from build123d import *

# Parameters (mm, degrees)
SKICA1_R               = 1.6
Z_KLADN_PLECH1_DEPTH   = 0.35
OHYB_START             = -2
OHYB_ZE_SKICI1_DEPTH   = 4
OHYB_ZE_SKICI1_2_DEPTH = 4


# Read off the part's stored shape, not the designer's step: Ohyb ze skici1
# Sheet-metal steps are written as plain solids
with BuildPart() as part:
    # Skica1 → Základní plech1 (new body)
    with BuildSketch(Plane(origin=(0, 0, 0), x_dir=(1, 0, 0), z_dir=(0, 1, 0))):
        with BuildLine():
            Line((6, 2), (13, 2))
            Line((13, 2), (13, -2))
            Line((13, -2), (6, -2))
            ThreePointArc((6, -2), (4.881966011, -2.263932023), (4, -3))
            ThreePointArc((4, -3), (-5, 0), (4, 3))
            ThreePointArc((4, 3), (4.881966011, 2.263932023), (6, 2))
        make_face()
        with Locations(Location((0, 0, 0), (0, 0, 270))):
            Circle(SKICA1_R, mode=Mode.SUBTRACT)
    extrude(amount=Z_KLADN_PLECH1_DEPTH)

    # Ohyb ze skici1 outline → Ohyb ze skici1 (cut)
    with BuildSketch(Plane.XY.offset(OHYB_START)):
        with BuildLine():
            ThreePointArc((7.3, 0.350000005), (7.728660709, 0.258514479), (8.082623799, 0))
            Line((8.082623799, 0), (13, 0))
            Line((13, 0), (13, 0.35))
            Line((13, 0.35), (7.3, 0.350000005))
        make_face()
    extrude(amount=OHYB_ZE_SKICI1_DEPTH, mode=Mode.SUBTRACT)

    # Ohyb ze skici1 2 outline → Ohyb ze skici1 2 (add)
    with BuildSketch(Plane.XY.offset(OHYB_START)):
        with BuildLine():
            Line((8.35, -5.025553214), (8.350000005, -0.700000005))
            ThreePointArc((8.350000005, -0.700000005), (8.280880984, -0.325336808), (8.082623799, 0))
            Line((8.082623799, 0), (7.3, 5e-09))
            ThreePointArc((7.3, 5e-09), (7.79497475, -0.20502525), (8.000000005, -0.7))
            Line((8.000000005, -0.7), (8, -5.025553214))
            Line((8, -5.025553214), (8.35, -5.025553214))
        make_face()
    extrude(amount=OHYB_ZE_SKICI1_2_DEPTH)


solid = part.part
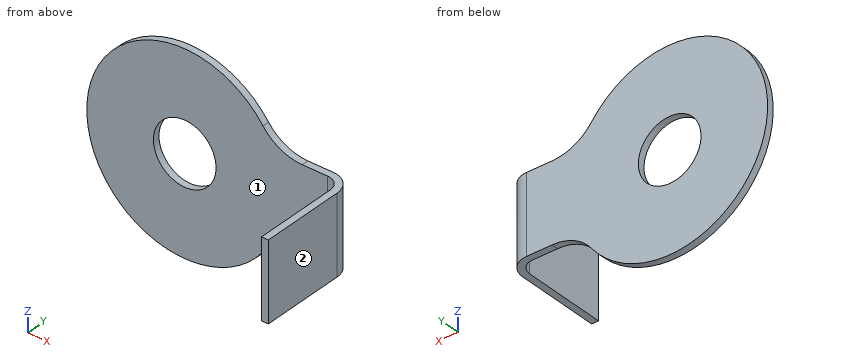
CAD build for the part. Positions are in the model's coordinates, mm. Face numbers are marked on the shaded views. A direction names the side the tool comes from. Round coordinates to 2 decimals unless told otherwise and drop trailing zeros. Order: outer loops, then holes, each group sorted by start corner. A loop starts at its lowest first (then second) coordinate and runs counter-clockwise, first axis right, second up. Notation, with made-up numbers: (-32.5, 3) - (-26.5, 3) arc R25 ccw to (-26.5, 23) - close; hole circle Ø5 at (-25.5, 39.25). An arc over 180 degrees is marked (long way). Return JSON: item names as keys, results as strings.
(1) Wall check: probe 1 along Y at (x, z) = (-0.75, 2); probe 2 along X at (y, z) = (0.25, 0); probe 3 along Z at (x, y) = (-0.5, 0.05). Give the ranges that are in metal, low to high. Write a range as from..to.
Answer key:
{"probe 1": "y = 0..0.35", "probe 2": "x = -5..-1.6, 1.6..7.75", "probe 3": "z = -4.97..-1.52, 1.52..4.97"}
(2) Cut at B-B (z = 0). Give the cut face in (x, y), then the cut area to 3 significant figures.
Answer key:
{"outline": "(-5, 0) - (-1.6, 0) - (-1.6, 0.35) - (-5, 0.35) - close; (1.6, 0) - (7.3, 0) arc R0.7 cw to (8, -0.7) - (8, -5.03) - (8.35, -5.03) - (8.35, -0.7) arc R1.05 ccw to (7.3, 0.35) - (1.6, 0.35) - close", "area": "5.18 mm^2"}
(3) Pin check, flat tips, straight feed: pin 1 Ø1 at (y, z) = (-2.5, 0.5) entering from -X; pin 2 Ø5 at (x, z) = (0, 0) entering from -Y; pin 3 Ø0.7 at (x, y) = (7, -3) entering from +Z; pin 4 Ø2.5 at (x, y) = (7.5, -2) entering from -Z. Stop position of each tip, or through.
Answer key:
{"pin 1": "stops at x = 8", "pin 2": "stops at y = 0", "pin 3": "passes through", "pin 4": "stops at z = -2"}
(4) Tool access for the marked faces 1 and 2: list every direction of +Z, -Z, +X, -X, +Y, -Y with a clear straight run to the whole face (end or side of a thin tool).
Answer key:
{"face 1": "+Z, -Z, -X, -Y", "face 2": "+Z, -Z, +X, +Y, -Y"}
(5) Cut at A-A (x = 0). Give the cut face in (y, z), then the cut area to 3 significant figures.
Answer key:
{"outline": "(0, -5) - (0.35, -5) - (0.35, -1.6) - (0, -1.6) - close; (0, 1.6) - (0.35, 1.6) - (0.35, 5) - (0, 5) - close", "area": "2.38 mm^2"}
(6) Cut at C-C (y = -1.8). Give the cut face in (x, z), then the cut area to 3 significant figures.
Answer key:
{"outline": "(8, -2) - (8.35, -2) - (8.35, 2) - (8, 2) - close", "area": "1.40 mm^2"}
(7) Cut at D-D (x = 3). Give the cut face in (y, z), then the cut area to 3 significant figures.
Answer key:
{"outline": "(0, -4) - (0.35, -4) - (0.35, 4) - (0, 4) - close", "area": "2.80 mm^2"}
